```python
from build123d import *

# Parameters (mm, degrees)
SKETCH1_W           = 266.7
SKETCH1_H           = 254
BOSS_EXTRUDE1_DEPTH = 4.826
SKETCH2_W           = 26.00000007
SKETCH2_H           = 82.55
CUT_EXTRUDE1_DEPTH  = 4.826
CUT_EXTRUDE3_DEPTH  = 4.826
SKETCH7_W           = 107.95
SKETCH7_H           = 25.4
CUT_EXTRUDE5_DEPTH  = 4.826
FILLET9_R           = 22.86
FILLET10_R          = 22.86
CUT_EXTRUDE6_DEPTH  = 4.826
SKETCH9_R           = 3.175
CUT_EXTRUDE7_DEPTH  = 4.826
SKETCH10_W          = 4.826
SKETCH10_H          = 16.51
CUT_EXTRUDE8_DEPTH  = 185.213226387
SKETCH12_W          = 4.826
SKETCH12_H          = 16.51
CUT_EXTRUDE9_DEPTH  = 185.213226387
SKETCH13_W          = 4.826
SKETCH13_H          = 16.51
CUT_EXTRUDE10_DEPTH = 185.213226387
SKETCH15_R          = 1.3462
CUT_EXTRUDE11_DEPTH = 185.213226387
SKETCH16_R          = 2.778125
SKETCH16_R_2        = 20.6375
CUT_EXTRUDE12_DEPTH = 185.213226387
SKETCH17_W          = 9.906
SKETCH17_H          = 5.588
CUT_EXTRUDE13_DEPTH = 185.213226387
SKETCH18_W          = 9.906
SKETCH18_H          = 5.588
CUT_EXTRUDE14_DEPTH = 185.213226387
SKETCH19_R          = 3.175
CUT_EXTRUDE15_DEPTH = 185.213226387
SKETCH20_R          = 1.905
CUT_EXTRUDE16_DEPTH = 185.213226387
SKETCH21_R          = 1.905
CUT_EXTRUDE17_DEPTH = 185.213226387


with BuildPart() as part:
    # Sketch1 → Boss-Extrude1 (new body)
    with BuildSketch(Plane(origin=(0, 0, 0), x_dir=(1, 0, 0), z_dir=(0, 1, 0))):
        Rectangle(SKETCH1_W, SKETCH1_H)
    extrude(amount=BOSS_EXTRUDE1_DEPTH)

    # Sketch2 → Cut-Extrude1 (cut)
    with BuildSketch(Plane(origin=(0, 4.826, 0), x_dir=(1, 0, 0), z_dir=(0, 1, 0))):
        with Locations((-120.349999965, -60.325)):
            Rectangle(SKETCH2_W, SKETCH2_H)
        with Locations((120.349999965, -60.325)):
            Rectangle(SKETCH2_W, SKETCH2_H)
    extrude(amount=-CUT_EXTRUDE1_DEPTH, mode=Mode.SUBTRACT)

    # Sketch4 → Cut-Extrude3 (cut)
    with BuildSketch(Plane(origin=(0, 4.826, 0), x_dir=(1, 0, 0), z_dir=(0, 1, 0))):
        with BuildLine():
            Line((-133.35, 101.6), (-133.35, 127))
            Line((-133.35, 127), (-107.95, 127))
            ThreePointArc((-107.95, 127), (-125.910512242, 119.560512242), (-133.35, 101.6))
        make_face()
        with BuildLine():
            Line((133.35, 101.6), (133.35, 127))
            Line((133.35, 127), (107.95, 127))
            ThreePointArc((107.95, 127), (125.910512242, 119.560512242), (133.35, 101.6))
        make_face()
    extrude(amount=-CUT_EXTRUDE3_DEPTH, mode=Mode.SUBTRACT)

    # Sketch7 → Cut-Extrude5 (cut)
    with BuildSketch(Plane(origin=(0, 4.826, 0), x_dir=(1, 0, 0), z_dir=(0, 1, 0))):
        with Locations((-53.975, 114.3)):
            Rectangle(SKETCH7_W, SKETCH7_H)
        with Locations((53.975, 114.3)):
            Rectangle(SKETCH7_W, SKETCH7_H)
    extrude(amount=-CUT_EXTRUDE5_DEPTH, mode=Mode.SUBTRACT)

    # Fillet9
    fillet9_edges = [part.edges().sort_by_distance(p)[0] for p in [
        (-107.95, 2.413, -101.6),
    ]]
    fillet(fillet9_edges, radius=FILLET9_R)

    # Fillet10
    fillet10_edges = [part.edges().sort_by_distance(p)[0] for p in [
        (107.95, 2.413, -101.6),
    ]]
    fillet(fillet10_edges, radius=FILLET10_R)

    # Sketch8 → Cut-Extrude6 (cut)
    with BuildSketch(Plane(origin=(0, 4.826, 0), x_dir=(1, 0, 0), z_dir=(0, 1, 0))):
        with BuildLine():
            Line((-133.35, -101.6), (-133.35, -127))
            Line((-133.35, -127), (-107.95, -127))
            ThreePointArc((-107.95, -127), (-125.910512242, -119.560512242), (-133.35, -101.6))
        make_face()
        with BuildLine():
            Line((133.35, -127), (107.95, -127))
            ThreePointArc((107.95, -127), (125.910512242, -119.560512242), (133.35, -101.6))
            Line((133.35, -101.6), (133.35, -127))
        make_face()
    extrude(amount=-CUT_EXTRUDE6_DEPTH, mode=Mode.SUBTRACT)

    # Sketch9 → Cut-Extrude7 (cut)
    with BuildSketch(Plane(origin=(0, 4.826, 0), x_dir=(1, 0, 0), z_dir=(0, 1, 0))):
        with Locations(Location((-71.12, -121.629004431, 0), (0, 0, 270))):
            Circle(SKETCH9_R)
        with Locations(Location((71.12, -121.629004431, 0), (0, 0, 90))):
            Circle(SKETCH9_R)
    extrude(amount=-CUT_EXTRUDE7_DEPTH, mode=Mode.SUBTRACT)

    # Sketch10 → Cut-Extrude8 (cut, through all)
    with BuildSketch(Plane(origin=(0, 4.826, 0), x_dir=(1, 0, 0), z_dir=(0, 1, 0))):
        with Locations((-104.93699993, -76.835)):
            Rectangle(SKETCH10_W, SKETCH10_H)
        with Locations((104.93699993, -43.815)):
            Rectangle(SKETCH10_W, SKETCH10_H)
        with Locations((104.93699993, -76.835)):
            Rectangle(SKETCH10_W, SKETCH10_H)
        with Locations((-104.93699993, -43.815)):
            Rectangle(SKETCH10_W, SKETCH10_H)
    extrude(amount=-CUT_EXTRUDE8_DEPTH, mode=Mode.SUBTRACT)

    # Sketch12 → Cut-Extrude9 (cut, through all)
    with BuildSketch(Plane.XZ):
        with Locations((-67.34499993, 76.835)):
            Rectangle(SKETCH12_W, SKETCH12_H)
        with Locations((-67.34499993, 43.815)):
            Rectangle(SKETCH12_W, SKETCH12_H)
    extrude(amount=-CUT_EXTRUDE9_DEPTH, mode=Mode.SUBTRACT)

    # Sketch13 → Cut-Extrude10 (cut, through all)
    with BuildSketch(Plane(origin=(0, 4.826, 0), x_dir=(1, 0, 0), z_dir=(0, 1, 0))):
        with Locations((67.34499993, -76.835)):
            Rectangle(SKETCH13_W, SKETCH13_H)
        with Locations((67.34499993, -43.815)):
            Rectangle(SKETCH13_W, SKETCH13_H)
    extrude(amount=-CUT_EXTRUDE10_DEPTH, mode=Mode.SUBTRACT)

    # Sketch15 → Cut-Extrude11 (cut, through all)
    with BuildSketch(Plane(origin=(0, 4.826, 0), x_dir=(1, 0, 0), z_dir=(0, 1, 0))):
        with Locations(Location((19.5961, -22.730838906, 0), (0, 0, 270))):
            Circle(SKETCH15_R)
        with Locations(Location((-19.6723, -22.730838906, 0), (0, 0, 270))):
            Circle(SKETCH15_R)
        with Locations(Location((-19.6723, -72.163561094, 0), (0, 0, 270))):
            Circle(SKETCH15_R)
        with Locations(Location((19.5961, -72.163561094, 0), (0, 0, 270))):
            Circle(SKETCH15_R)
    extrude(amount=-CUT_EXTRUDE11_DEPTH, mode=Mode.SUBTRACT)

    # Sketch16 → Cut-Extrude12 (cut, through all)
    with BuildSketch(Plane(origin=(0, 4.826, 0), x_dir=(1, 0, 0), z_dir=(0, 1, 0))):
        with Locations(Location((77.293854564, 60.610218612, 0), (0, 0, 270))):
            Circle(SKETCH16_R)
        with Locations(Location((114.3, 19.164632523, 0), (0, 0, 270))):
            Circle(SKETCH16_R)
        with Locations(Location((95.796927282, 39.887425568, 0), (0, 0, 270))):
            Circle(SKETCH16_R_2)
        with Locations(Location((-95.796927282, 39.887425568, 0), (0, 0, 90))):
            Circle(SKETCH16_R_2)
        with Locations(Location((-77.293854564, 60.610218612, 0), (0, 0, 90))):
            Circle(SKETCH16_R)
        with Locations(Location((-114.3, 19.164632523, 0), (0, 0, 90))):
            Circle(SKETCH16_R)
    extrude(amount=-CUT_EXTRUDE12_DEPTH, mode=Mode.SUBTRACT)

    # Sketch17 → Cut-Extrude13 (cut, through all)
    with BuildSketch(Plane(origin=(0, 4.826, 0), x_dir=(1, 0, 0), z_dir=(0, 1, 0))):
        with Locations((-67.795869789, 77.244822677)):
            Rectangle(SKETCH17_W, SKETCH17_H)
        with Locations((-105.895869789, 77.244822677)):
            Rectangle(SKETCH17_W, SKETCH17_H)
        with Locations((-29.695869789, 77.244822677)):
            Rectangle(SKETCH17_W, SKETCH17_H)
        with Locations((29.695869789, 77.244822677)):
            Rectangle(SKETCH17_W, SKETCH17_H)
        with Locations((67.795869789, 77.244822677)):
            Rectangle(SKETCH17_W, SKETCH17_H)
        with Locations((105.895869789, 77.244822677)):
            Rectangle(SKETCH17_W, SKETCH17_H)
        with Locations((0, 77.244822677)):
            Rectangle(SKETCH17_W, SKETCH17_H)
    extrude(amount=-CUT_EXTRUDE13_DEPTH, mode=Mode.SUBTRACT)

    # Sketch18 → Cut-Extrude14 (cut, through all)
    with BuildSketch(Plane(origin=(0, 4.826, 0), x_dir=(1, 0, 0), z_dir=(0, 1, 0))):
        with Locations((0, -101.6)):
            Rectangle(SKETCH18_W, SKETCH18_H)
        with Locations((0, -81.28)):
            Rectangle(SKETCH18_W, SKETCH18_H)
    extrude(amount=-CUT_EXTRUDE14_DEPTH, mode=Mode.SUBTRACT)

    # Sketch19 → Cut-Extrude15 (cut, through all)
    with BuildSketch(Plane(origin=(0, 4.826, 0), x_dir=(1, 0, 0), z_dir=(0, 1, 0))):
        with Locations(Location((0, 55.982011538, 0), (0, 0, 270))):
            Circle(SKETCH19_R)
        with Locations(Location((12.7, 55.982011538, 0), (0, 0, 270))):
            Circle(SKETCH19_R)
        with Locations(Location((-12.7, 55.982011538, 0), (0, 0, 270))):
            Circle(SKETCH19_R)
    extrude(amount=-CUT_EXTRUDE15_DEPTH, mode=Mode.SUBTRACT)

    # Sketch20 → Cut-Extrude16 (cut, through all)
    with BuildSketch(Plane(origin=(0, 4.826, 0), x_dir=(1, 0, 0), z_dir=(0, 1, 0))):
        with Locations(Location((-17.603854564, 38.202011538, 0), (0, 0, 270))):
            Circle(SKETCH20_R)
        with Locations(Location((-58.243854564, 38.202011538, 0), (0, 0, 270))):
            Circle(SKETCH20_R)
        with Locations(Location((-58.243854564, -12.597988462, 0), (0, 0, 270))):
            Circle(SKETCH20_R)
        with Locations(Location((-17.603854564, -12.597988462, 0), (0, 0, 270))):
            Circle(SKETCH20_R)
    extrude(amount=-CUT_EXTRUDE16_DEPTH, mode=Mode.SUBTRACT)

    # Sketch21 → Cut-Extrude17 (cut, through all)
    with BuildSketch(Plane(origin=(0, 4.826, 0), x_dir=(1, 0, 0), z_dir=(0, 1, 0))):
        with Locations(Location((7.796145436, 28.154731738, 0), (0, 0, 270))):
            Circle(SKETCH21_R)
        with Locations(Location((58.596145436, 28.154731738, 0), (0, 0, 270))):
            Circle(SKETCH21_R)
        with Locations(Location((7.796145436, -12.485268262, 0), (0, 0, 270))):
            Circle(SKETCH21_R)
        with Locations(Location((58.596145436, -12.485268262, 0), (0, 0, 270))):
            Circle(SKETCH21_R)
    extrude(amount=-CUT_EXTRUDE17_DEPTH, mode=Mode.SUBTRACT)


solid = part.part
```
Here's how the part is built. I have some questions about the finished solid (model axes, mm). A direction names the side the tool comes from. Coordinates: 2 decimals unless noted, no trailing zeros. Write each loop counter-clockwise with the first axis right and the second up, starting at its lowest first coordinate (ties: lowest second). Pieces come first, ordered by that corner, then holes. Notation, with made-up numbers: (26.5, 84) -> (44.5, 84) arc R22 ccw to (44.5, 107) -> close; hole circle Ø3 at (-13, -11). An arc over 180 degrees is marked (long way). Use a Markdown table: item, result. Add a question column.
(1) Please list where these lines run through material, in increasing order: line 1 (X direction, y = 3.25, z = 43); line 2 (Z direction, x = -0.5, y = 3.1); line 3 (Z direction, x = 114.5, y = 4.1).
(2) If we section it at C-C, the plane x = -43: Write out the boundary of the cut face in (y, z).
(3) If we section it at A-A, the plane x = -12.7: Write out the boundary of the cut face in (y, z), and give its area (3 significant figures).
(4) If we section it at B-B, the plane z = 94.5: Write out the boundary of the cut face in (x, y), and give its area (3 significant figures).
(5) For faces 4 (the cylindrical face through (-101.431, 2.379, -108.474)), 5 (the cylindrical face through (125.71, 2.45, -119.76)), which set-ups out of +Z, -Z, +X, -X, +Y, -Y let a thin tool reach every point of the face, with its end or its side?
(6) We'd pull the mould along Z, two halves only. Please class faces 1 (the cylindrical face through (75.6, 2.45, -62.81)), 2 (the flat face through (-2, 4.826, -2)), 3 (the cylindrical face through (101.076, 2.379, -108.119)): +Z half, -Z half, draft (parallel to the pull), parting line (faces both ways), or undercut.
(7) If we section it at D-D, the plane y = 0.9: State how many separate pieces and enclosed holes the cut face has, and give its area (3 significant figures).
(8) I'm going to push flat-ended pins straight in: P1, Ø1.4, axis at y = 2.5, z = 77, coming from the -X side; P2, Ø3.5, axis at x = -17.6, z = 12.6, coming from the +Y side; P3, Ø1.5, axis at y = 1.5, z = 64, coming from the +X side; P4, Ø2, axis at x = 105, y = 1, coming from the -Z side. Where does each tip first touch, or does it pass through?
Outcome:
| question | item | result |
|---|---|---|
| 1 | line 1 | x = -102.52 to -69.76, -64.93 to 64.93, 69.76 to 102.52 |
| 1 | line 2 | z = -101.6 to -80.04, -74.45 to -59.12, -52.85 to 78.49, 84.07 to 98.81, 104.39 to 127 |
| 1 | line 3 | z = -126.14 to -48.61, -31.16 to -21.94, -16.39 to 19.05, 101.6 to 126.14 |
| 2 | outline | (0, -101.6) -> (4.83, -101.6) -> (4.83, 127) -> (0, 127) -> close |
| 3 | outline | (0, -101.6) -> (4.83, -101.6) -> (4.83, -59.16) -> (0, -59.16) -> close; (0, -52.81) -> (4.83, -52.81) -> (4.83, 127) -> (0, 127) -> close |
| 3 | area | 1,070 mm^2 |
| 4 | outline | (-107.35, 0) -> (107.35, 0) -> (107.35, 4.83) -> (-107.35, 4.83) -> close |
| 4 | area | 1,040 mm^2 |
| 5 | face 4 | -Z, +Y, -Y |
| 5 | face 5 | -Z, +X, +Y, -Y |
| 6 | face 1 | undercut |
| 6 | face 2 | draft |
| 6 | face 3 | -Z half |
| 7 | separate pieces | 1 |
| 7 | enclosed holes | 36 |
| 7 | area | 53,500 mm^2 |
| 8 | P1 | stops at x = -102.52 |
| 8 | P2 | passes through |
| 8 | P3 | stops at x = 107.35 |
| 8 | P4 | stops at z = -115.22 |
